from build123d import *

# Parameters (mm, degrees)
SKETCH1_R           = 4.09575
SKETCH1_R_2         = 1.651
BOSS_EXTRUDE1_DEPTH = 3.175
CUT_EXTRUDE2_DEPTH  = 6.35
SKETCH7_R           = 4.9784
SKETCH7_R_2         = 1.5875
CUT_EXTRUDE3_DEPTH  = 124.96234811
FILLET1_R           = 6.35
SKETCH8_W           = 50.8
SKETCH8_H           = 12.7
CUT_EXTRUDE4_DEPTH  = 50.8
CUT_EXTRUDE5_DEPTH  = 19.304
FILLET6_R           = 6.35
FILLET7_R           = 6.35
FILLET8_R           = 19.05
BOSS_EXTRUDE2_DEPTH = 3.175
FILLET9_R           = 24.13
SKETCH13_W          = 50.8
SKETCH13_H          = 9.69768102
SKETCH13_W_2        = 38.1
SKETCH13_H_2        = 8.504610511
BOSS_EXTRUDE3_DEPTH = 6.35


with BuildPart() as part:
    # Sketch1 → Boss-Extrude1 (new body)
    with BuildSketch(Plane.XY):
        with BuildLine():
            Line((0, 0), (107.95, 0))
            Line((107.95, 0), (100.9362606, 26.175631792))
            Line((100.9362606, 26.175631792), (100.868755024, 26.427566033))
            ThreePointArc((100.868755024, 26.427566033), (110.348359368, 43.438223217), (95.367453293, 55.88))
            Line((95.367453293, 55.88), (0, 38.1))
            Line((0, 38.1), (0, 25.4))
            Line((0, 25.4), (-7.62, 25.4))
            Line((-7.62, 25.4), (-7.62, 12.7))
            Line((-7.62, 12.7), (0, 12.7))
            Line((0, 12.7), (0, 0))
        make_face()
        with Locations((95.367453293, 40.64)):
            Circle(SKETCH1_R, mode=Mode.SUBTRACT)
        with Locations((25.817011896, 25.817011896)):
            Circle(SKETCH1_R_2, mode=Mode.SUBTRACT)
        with Locations((25.817011896, 12.282988104)):
            Circle(SKETCH1_R_2, mode=Mode.SUBTRACT)
        with Locations((12.282988104, 12.282988104)):
            Circle(SKETCH1_R_2, mode=Mode.SUBTRACT)
        with Locations((12.282988104, 25.817011896)):
            Circle(SKETCH1_R_2, mode=Mode.SUBTRACT)
    extrude(amount=BOSS_EXTRUDE1_DEPTH)

    # Sketch6 → Cut-Extrude2 (cut)
    with BuildSketch(Plane.XY.offset(3.175)):
        with BuildLine():
            Line((50.8, 0), (76.2, 0))
            ThreePointArc((76.2, 0), (63.5, 12.7), (50.8, 0))
        make_face()
    extrude(amount=-CUT_EXTRUDE2_DEPTH, mode=Mode.SUBTRACT)

    # Sketch7 → Cut-Extrude3 (cut, through all)
    with BuildSketch(Plane.XY.offset(3.175)):
        with Locations((19.05, 19.05)):
            Circle(SKETCH7_R)
        with Locations((80.766582748, 12.282988104)):
            Circle(SKETCH7_R_2)
        with Locations((94.299702748, 12.282988104)):
            Circle(SKETCH7_R_2)
        with Locations((80.766582748, 25.817011896)):
            Circle(SKETCH7_R_2)
        with Locations((94.299702748, 25.817011896)):
            Circle(SKETCH7_R_2)
    extrude(amount=-CUT_EXTRUDE3_DEPTH, mode=Mode.SUBTRACT)

    # Fillet1
    fillet1_edges = [part.edges().sort_by_distance(p)[0] for p in [
        (100.868755024, 26.427566033, 1.5875),
    ]]
    fillet(fillet1_edges, radius=FILLET1_R)

    # Sketch8 → Cut-Extrude4 (cut)
    with BuildSketch(Plane.XY.offset(3.175)):
        with Locations((25.4, 44.45)):
            Rectangle(SKETCH8_W, SKETCH8_H)
    extrude(amount=-CUT_EXTRUDE4_DEPTH, mode=Mode.SUBTRACT)

    # Sketch9 → Cut-Extrude5 (cut)
    with BuildSketch(Plane.XY.offset(3.175)):
        Polygon((50.8, 47.57098794), (50.8, 40.64), (57.15, 40.64), (57.15, 48.754861432), align=None)
    extrude(amount=-CUT_EXTRUDE5_DEPTH, mode=Mode.SUBTRACT)

    # Fillet6
    fillet6_edges = [part.edges().sort_by_distance(p)[0] for p in [
        (57.15, 40.64, 1.5875),
    ]]
    fillet(fillet6_edges, radius=FILLET6_R - 0.0001)  # a hair under: the kernel refuses the full size

    # Fillet7
    fillet7_edges = [part.edges().sort_by_distance(p)[0] for p in [
        (57.15, 48.754861432, 1.5875),
    ]]
    fillet(fillet7_edges, radius=FILLET7_R)

    # Fillet8
    fillet8_edges = [part.edges().sort_by_distance(p)[0] for p in [
        (50.8, 0, 1.5875),
    ]]
    fillet(fillet8_edges, radius=FILLET8_R)

    # Sketch12 → Boss-Extrude2 (add)
    with BuildSketch(Plane.XY.offset(3.175)):
        with BuildLine():
            Line((50.8, 40.64), (85.027112904, 40.64))
            Line((85.027112904, 40.64), (95.367453293, 55.88))
            add(Edge.make_bspline(
                [(50.8, 40.64), (70.777788932, 52.178803671), (78.594281742, 111.543427795), (95.367453293, 55.88)],
                knots=[0, 0, 0, 0, 1, 1, 1, 1], degree=3))
        make_face()
    extrude(amount=-BOSS_EXTRUDE2_DEPTH)

    # Fillet9
    fillet9_edges = [part.edges().sort_by_distance(p)[0] for p in [
        (95.367453293, 55.88, 1.5875),
    ]]
    fillet(fillet9_edges, radius=FILLET9_R)

    # Sketch13 → Boss-Extrude3 (add)
    with BuildSketch(Plane(origin=(0, 0, 0), x_dir=(-1, 0, 0), z_dir=(0, 0, -1))):
        with Locations((-25.4, 33.25115949)):
            Rectangle(SKETCH13_W, SKETCH13_H)
        with Locations((-19.05, 4.252305256)):
            Rectangle(SKETCH13_W_2, SKETCH13_H_2)
    extrude(amount=-BOSS_EXTRUDE3_DEPTH)


solid = part.part
Can you work these out from the model? Positions are in its coordinate system, mm. A direction names the side the tool comes from. Round coordinates to 2 decimals unless told otherwise and drop trailing zeros. Order: outer loops, then holes, each group sorted by start corner. A loop starts at its lowest first (then second) coordinate and runs counter-clockwise, first axis right, second up. Notation, with made-up numbers: M -31.5,23.25 L 8.5,23.25 A28 cw 8.5,50.25 Z; hole C -24.75,31 d7. An arc over 180 degrees is marked long. Use a Markdown table: item, result.
1) Imagine slicing it at B-B (y = 19.05). List the corners of the cut face in (x, z) for me (3 decimals), then the cut area to 3 significant figures.
Geometry says:
| item | result |
|---|---|
| outline | M -7.62,0 L 14.072,0 L 14.072,3.175 L -7.62,3.175 Z; M 24.028,0 L 102.846,0 L 102.846,3.175 L 24.028,3.175 Z |
| area | 319 mm² |
2) Imagine slicing it at A-A (x = 19.05). List the corners of the cut face in (y, z) for me (3 decimals), then the cut area to 3 significant figures.
Geometry says:
| item | result |
|---|---|
| outline | M 0,0 L 14.072,0 L 14.072,3.175 L 8.505,3.175 L 8.505,6.35 L 0,6.35 Z; M 24.028,0 L 38.1,0 L 38.1,6.35 L 28.402,6.35 L 28.402,3.175 L 24.028,3.175 Z |
| area | 147 mm² |
3) I'm going to push flat-ended pins straight in: P1, Ø4, axis at x = 92.5, y = 59.5, coming from the +Z side (3 decimals); P2, Ø1.6, axis at x = -3.5, z = 2, coming from the +Y side; P3, Ø5.5, axis at x = 25.82, y = 25.82, coming from the -Z side; P4, Ø2.5, axis at x = 94.3, y = 12.28, coming from the -Z side. Where does each tip first touch, or does it pass through?
Geometry says:
| item | result |
|---|---|
| P1 | stops at z = 3.175 |
| P2 | stops at y = 25.4 |
| P3 | stops at z = 0 |
| P4 | passes through |
4) If I drill on line 1 along Y through (x, z) = (19.5, 2.5); line 2 along Y through (x, z) = (1.5, 1.5); line 3 along Y through (x, z) = (26, 3.25), over which ranges is the centre line in solid material (lowest first)?
Geometry says:
| item | result |
|---|---|
| line 1 | y = 0 to 14.09, 24.01 to 38.1 |
| line 2 | y = 0 to 38.1 |
| line 3 | y = 0 to 8.5, 28.4 to 38.1 |
5) Imagine slicing it at C-C (x = 46). List the corners of the cut face in (y, z) for me (3 decimals), then the cut area to 3 significant figures.
Geometry says:
| item | result |
|---|---|
| outline | M 1.715,0 L 38.1,0 L 38.1,6.35 L 28.402,6.35 L 28.402,3.175 L 1.715,3.175 Z |
| area | 146 mm² |
6) Imagine slicing it at D-D (z = 1). Give the number of separate pieces and of enclosed holes in the cut face, then the cut area to 3 significant figures.
Geometry says:
| item | result |
|---|---|
| separate pieces | 1 |
| enclosed holes | 10 |
| area | 5,020 mm² |
7) On a 3-axis mill with a long thin cutter (end or side, diameter ignored), from which of +Z, -Z, +X, -X, +Y, -Y can I reach the whole of each face in a straight line? I mean faces 1 (the face through (95.032, 24.409, 1.61)), 2 (the face through (-4, 12.7, 2)), 3 (the face through (50.8, 39, 2)), 4 (the face through (26, 28.402, 5)), 5 (the face through (38.1, 4, 5)). Say none if no direction works.
Geometry says:
| item | result |
|---|---|
| face 1 | +Z, -Z |
| face 2 | +Z, -Z, -X, -Y |
| face 3 | +Z, -Z, -X, +Y |
| face 4 | +Z, +X, -X |
| face 5 | +Z, +X, -Y |
